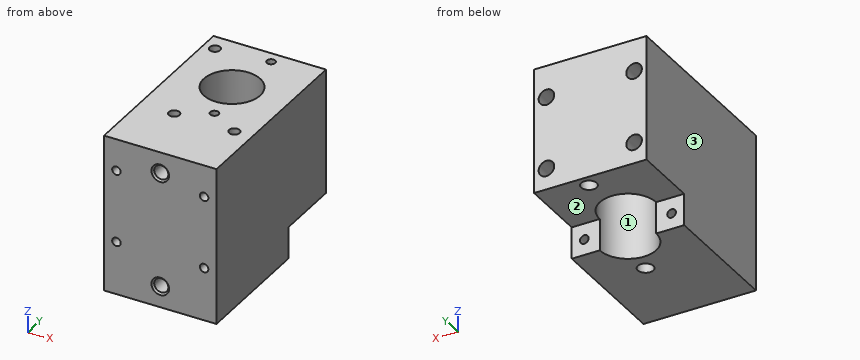
Autodesk Inventor part; units mm, degrees
ref_plane "YZ Plane" through (0, 0, 0) normal (1, 0, 0) x (0, 1, 0)
ref_plane "XZ Plane" through (0, 0, 0) normal (0, 1, 0) x (-1, 0, 0)
ref_plane "XY Plane" through (0, 0, 0) normal (0, 0, 1) x (1, 0, 0)
sketch "Sketch1" plane through (0, 0, 0) normal (0, 0, 1) x (1, 0, 0)
  line L0 (-15.875, 18.975) -> (15.875, 18.975)
  line L1 (15.875, 18.975) -> (15.875, -35)
  line L2 (15.875, -35) -> (-15.875, -35)
  line L3 (-15.875, -35) -> (-15.875, 18.975)
  point P0 (0, 0)
  dimension "d0" = 31.75
  dimension "d1" = 53.975
  dimension "d3" = 35
  dimension "d4" = 15.875
extrude "Extrusion1" add sketch "Sketch1" along normal blind 44.45
sketch "Sketch2" plane through (0, 0, 44.45) normal (0, 0, 1) x (1, 0, 0)
  circle A0 centre (0, 0.3862) radius 7.9629
  line L0 (15.875, 18.975) -> (-15.875, 18.975)
  line L1 (-15.875, 18.975) -> (-15.875, -35)
  line L2 (-15.875, -35) -> (15.875, -35)
  line L3 (15.875, -35) -> (15.875, 18.975)
  line L4 (15.875, 18.975) -> (-15.875, 18.975)
  line L5 (0, 18.975) -> (0, -35) construction
  dimension "d7" = 15.9258
  dimension "d124" = 35.3862
extrude "Extrusion2" cut sketch "Sketch2" against normal through all contours A0
sketch "Sketch4" plane through (-15.875, 18.975, 0) normal (0, 1, 0) x (1, 0, 0)
  line L0 (0, 0) -> (31.75, 0)
  line L1 (31.75, 0) -> (0, 0)
  line L2 (0, 0) -> (0, -9)
  line L3 (0, -9) -> (31.75, -9)
  line L4 (31.75, -9) -> (31.75, 0)
  line L5 (0, 0) -> (0, -44.45)
  point P0 (15.875, 0)
  point P1 (0, -4.5)
  dimension "d15" = 9
extrude "Extrusion4" cut sketch "Sketch4" against normal blind 18.5888
sketch "Sketch6" plane through (0, 0, 44.45) normal (0, 0, 1) x (1, 0, 0)
  line L0 (15.875, -15.95) -> (-11.125, -15.95)
  line L1 (-11.125, -15.95) -> (-11.125, 18.975)
  point P0 (0, 0)
  point P1 (-6.125, -17.45)
  point P2 (10.875, -17.45)
  point P3 (-12.625, 13.975)
  dimension "d33" = 1.5
  dimension "d34" = 1.5
  dimension "d35" = 5
  dimension "d36" = 5
  dimension "d44" = 5
  dimension "d45" = 1.5
hole "Press fit for D3mm_L10mm Dowel - pin to protrude 5mm" at (-6.125, -17.45, 44.45) at (10.875, -17.45, 44.45) at (-12.625, 13.975, 44.45) direction (0, 0, -1) diameter 3 depth 5 tip angle 118
sketch "Sketch9" plane through (-15.875, 18.975, 44.45) normal (0, 1, 0) x (1, 0, 0)
  line L0 (31.75, 35.45) -> (0, 35.45)
  line L1 (0, 35.45) -> (0, 0)
  line L2 (31.75, 0) -> (0, 0)
  line L3 (31.75, 35.45) -> (31.75, 0)
  line L4 (23.8379, 35.45) -> (23.8379, 44.45)
  line L5 (7.9121, 44.45) -> (23.8379, 44.45)
  line L6 (7.9121, 44.45) -> (7.9121, 35.45)
  line L7 (7.9121, 35.45) -> (23.8379, 35.45)
  line L8 (23.8379, 0) -> (7.9121, 0)
  point P0 (15.875, 44.45)
  point P1 (28.25, 9)
  point P2 (3.5, 9)
  point P3 (3.5, 29.45)
  point P4 (28.25, 29.45)
  dimension "d60" = 9
  dimension "d61" = 3.5
  dimension "d62" = 3.5
  dimension "d63" = 9
  dimension "d96" = 6
  dimension "d97" = 6
  dimension "d98" = 3.5
  dimension "d99" = 3.5
hole "Cbore hole for M2 screw_1" at (12.375, 18.975, 35.45) at (-12.375, 18.975, 35.45) at (-12.375, 18.975, 15) at (12.375, 18.975, 15) direction (0, -1, 0) diameter 2.4 end through all counterbore diameter 4.4 counterbore depth 39
sketch "Sketch11" plane through (15.875, 18.975, 9) normal (0, 0, -1) x (-1, 0, 0)
  circle A0 centre (13.5, -3.5) radius 0.7835
  point P0 (15.875, -18.975)
hole "Cbore hole for M2 screw_2" at (2.375, 15.475, 9) direction (0, 0, 1) diameter 2.4 end through all counterbore diameter 4.4 counterbore depth 20
sketch "Sketch12" plane through (0, 0, 0) normal (0, 0, -1) x (-1, 0, 0)
  circle A0 centre (-2.375, -12.45) radius 0.7835
  point P0 (0, 0)
hole "Cbore hole for M2 screw_3" at (2.375, -12.45, 0) direction (0, 0, 1) diameter 2.4 end through all counterbore diameter 4.4 counterbore depth 29
sketch "Sketch13" plane through (-15.875, -35, 0) normal (0, -1, 0) x (1, 0, 0)
  circle A0 centre (3.5, 15) radius 1.2
  circle A1 centre (28.25, 35.45) radius 1.2
  circle A2 centre (3.5, 35.45) radius 1.2
  circle A3 centre (28.25, 15) radius 1.2
  line L0 (31.75, 0) -> (0, 0)
  line L1 (31.75, 0) -> (31.75, 44.45)
  line L2 (0, 44.45) -> (31.75, 44.45)
  line L3 (0, 0) -> (0, 44.45)
  line L4 (0, 44.45) -> (31.75, 44.45)
  line L5 (20.45, 0) -> (16.05, 0)
  line L6 (15.875, 44.45) -> (15.875, 0) construction
  point P0 (15.875, 0)
  point P1 (15.875, 38.45)
  point P2 (15.875, 6)
  dimension "d100" = 6
  dimension "d101" = 6
hole "Locating Holes for Mitsumi CJPDB3-4" at (0, -35, 38.45) at (0, -35, 6) direction (0, 1, 0) diameter 4 depth 8 tip angle 118 countersink diameter 5 countersink angle 90
sketch "Sketch15" plane through (-15.875, 0.3862, 0) normal (0, 1, 0) x (1, 0, 0)
  circle A0 centre (3.556, -4.445) radius 1.7
  circle A1 centre (28.194, -4.445) radius 1.7
  point P0 (15.875, 0)
hole "Threaded hole for M3 screw" at (12.319, 0.3862, 4.445) at (-12.319, 0.3862, 4.445) direction (0, -1, 0) diameter 2.459 depth 10 tip angle 118
properties part number "J007515" material "ALUMINUM, 6061-T651"
Design review of the part built by this model. Coordinates are the model's own, in mm. Face numbers are marked on the shaded views. Give positions to 0.01 mm unless a question says otherwise; leave off trailing zeros. Write each loop counter-clockwise with the first axis right and the second up, starting at its lowest first coordinate (ties: lowest second). Pieces come first, ordered by that corner, then holes. Notation, with made-up numbers: M 67.25,-1 L 114.25,-1 A24 ccw 114.25,21 Z; hole C 55,27.25 d2. An arc over 180 degrees is marked long. Return JSON: item names as keys, results as strings. Group by question number.
Item 1: Take a section at B-B (z = 31). Give the boundary of the cut face in (x, y) (3 decimals), plus the area to 3 significant figures.
Item 2: Take a section at C-C (y = -12.45). Give the boundary of the cut face in (x, z) (3 decimals), plus the area to 3 significant figures.
Item 3: The part is to be moulded in two halves that separate along X. For the marked faces 1, 2 and 3, say which applies: pulls with the +X half, pulls with the -X half, needs draft (parallel to the pull), parting line crosses it, or undercut.
Item 4: Wall thickness on line 1 along X through (y, z) = (-32, 35.45) (3 decimals); line 2 along X through (y, z) = (0, 7) (3 decimals); line 3 along Z through (x, y) = (12, 13): over which ranges is each line inside the solid? List them lowest first.
Item 5: Take a section at D-D (y = -31). Give the boundary of the cut face in (x, z) (3 decimals), plus the area to 3 significant figures.
Item 6: Take a section at A-A (y = 5). Give the boundary of the cut face in (x, z) (3 decimals).
Item 7: Clearance check with flat-ended pins moving along their axes: pin 1 Ø3.5 at (x, z) = (-12.375, 35.45) entering from -Y; pin 2 Ø3.5 at (x, z) = (0, 6) entering from -Y; pin 3 Ø1.4 at (x, y) = (2.375, -12.45) entering from +Z; pin 4 Ø15 at (x, y) = (-4, 12) entering from -Z. State where each tip first meets the part, or that it passes through.
Return value:
{
 "1": {"outline": "M -15.875,-35 L 15.875,-35 L 15.875,18.975 L -15.875,18.975 Z; hole C 0,0.386 d15.926; hole C 2.375,-12.45 d2.4; hole C 2.375,15.475 d2.4", "area": "1,510 mm2"},
 "2": {"outline": "M -15.875,0 L 0.175,0 L 0.175,29 L 1.175,29 L 1.175,44.45 L -15.875,44.45 Z; M 3.575,29 L 4.575,29 L 4.575,0 L 15.875,0 L 15.875,44.45 L 3.575,44.45 Z; hole C -12.375,15 d4.4; hole C -12.375,35.45 d4.4; hole C 12.375,15 d4.4; hole C 12.375,35.45 d4.4", "area": "1,190 mm2"},
 "3": {"face 1": "undercut", "face 2": "needs draft", "face 3": "pulls with the -X half"},
 "4": {"line 1": "x = -15.875 to -13.575, -11.175 to 11.175, 13.575 to 15.875", "line 2": "x = -15.875 to -7.954, 7.954 to 15.875", "line 3": "z = 9 to 12.83, 17.17 to 33.28, 37.62 to 44.45"},
 "5": {"outline": "M -15.875,0 L 15.875,0 L 15.875,44.45 L -15.875,44.45 Z; hole C -12.375,15 d2.4; hole C -12.375,35.45 d2.4; hole C 0,6 d4; hole C 0,38.45 d4; hole C 12.375,15 d2.4; hole C 12.375,35.45 d2.4", "area": "1,370 mm2"},
 "6": {"outline": "M -15.875,9 L -6.49,9 L -6.49,44.45 L -15.875,44.45 Z; M 6.49,9 L 15.875,9 L 15.875,44.45 L 6.49,44.45 Z; hole C -12.375,15 d4.4; hole C -12.375,35.45 d4.4; hole C 12.375,15 d4.4; hole C 12.375,35.45 d4.4"},
 "7": {"pin 1": "stops at y = -35", "pin 2": "stops at y = -26.85", "pin 3": "passes through", "pin 4": "stops at z = 9"}
}
